Read the model definition and answer for the solid it produces. Units are mm, in the model's axes. Face numbers are marked on the shaded views. Coordinates: 2 decimals unless noted, no trailing zeros. Loops run counter-clockwise (first coordinate to the right, second up) from the corner with the lowest first, then second, coordinate; pieces in that order, holes last. Notation, with made-up numbers: M 69.5,9.5 L 124.5,9.5 A23 ccw 124.5,23.5 Z; hole C 59,-22 d6. An arc over 180 degrees is marked long. Put each result on its own line as item: value.
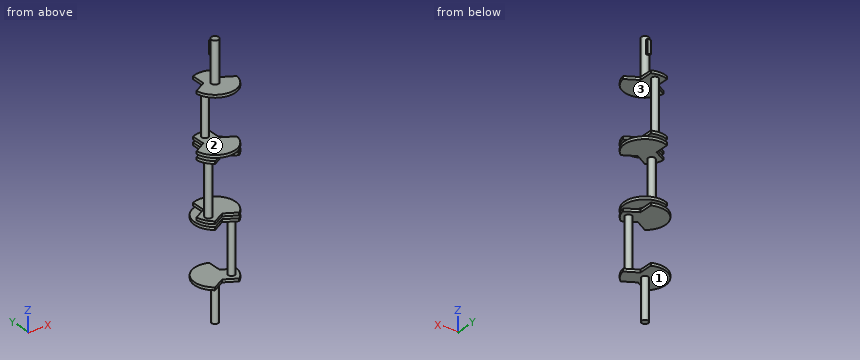
from build123d import *

# Parameters (mm, degrees)
BOSS_EXTRUDE1_DEPTH      = 5.08
LPATTERN1_COUNT          = 2
LPATTERN1_PITCH          = 104.14
BOSS_EXTRUDE2_REACH      = 119.176
SKETCH3_R                = 6.35
LPATTERN2_COUNT          = 3
LPATTERN2_PITCH          = 114.3
BODY_MOVE_COPY2_ANGLE    = 120
BODY_MOVE_COPY3_ANGLE    = 120
BOSS_EXTRUDE3_REACH      = 236.864
SKETCH5_R                = 12.7
BOSS_EXTRUDE4_START      = 114.3
SKETCH5_2_R              = 12.7
BOSS_EXTRUDE4_DEPTH      = 5.08
SKETCH6_R                = 6.985
BOSS_EXTRUDE5_DEPTH      = 76.2
SKETCH7_R                = 6.35
BOSS_EXTRUDE6_DEPTH      = 76.2
BOSS_EXTRUDE7_REACH      = 424.634
BOSS_EXTRUDE7_END_RADIUS = 6.985
BOSS_EXTRUDE7_START      = 10.16
SKETCH8_W                = 6.35
SKETCH8_H                = 25.4


with BuildPart() as part:
    # Sketch2 → Boss-Extrude1 (new body)
    with BuildSketch(Plane.XY):
        with BuildLine():
            Line((15.24, 8.798818102), (15.24, 34.919226796))
            ThreePointArc((15.24, 34.919226796), (0, 38.1), (-15.24, 34.919226796))
            Line((-15.24, 34.919226796), (-15.24, 8.798818102))
            Line((-15.24, 8.798818102), (-37.860937485, -4.261386244))
            ThreePointArc((-37.860937485, -4.261386244), (0, -38.1), (37.860937485, -4.261386244))
            Line((37.860937485, -4.261386244), (15.24, 8.798818102))
        make_face()
    extrude(amount=-BOSS_EXTRUDE1_DEPTH)


with BuildPart() as lpattern1_1:
    # LPattern1: pattern copy
    add(part.part.moved(Location(Vector(0, 0, 1) * (1 * LPATTERN1_PITCH))))

    # Sketch3 → Boss-Extrude2 (add, up to next)
    with BuildSketch(Plane.XY, mode=Mode.PRIVATE) as boss_extrude2_sk1:
        with Locations((0, 25.038762276)):
            Circle(SKETCH3_R)
    boss_extrude2_tool1 = extrude(boss_extrude2_sk1.sketch, amount=BOSS_EXTRUDE2_REACH, mode=Mode.PRIVATE) - lpattern1_1.part

    add(part.part)  # Boss-Extrude2 merges part
    add(boss_extrude2_tool1.solids().sort_by_distance((0, 25.038762, 0))[0])


with BuildPart() as lpattern2_1:
    # LPattern2: pattern copy
    add(lpattern1_1.part.moved(Location(Vector(0, 0, 1) * (1 * LPATTERN2_PITCH))))


with BuildPart() as lpattern2_2:
    # LPattern2: pattern copy
    add(lpattern1_1.part.moved(Location(Vector(0, 0, 1) * (2 * LPATTERN2_PITCH))))


with BuildPart() as lpattern2_1_1:
    # Body-Move/Copy2: moved
    add(lpattern2_1.part.rotate(Axis((0, -0.157266766, 0), (0, 0, 1)), BODY_MOVE_COPY2_ANGLE))

    # Sketch5 → Boss-Extrude3 (add, up to next)
    with BuildSketch(Plane.XY.offset(104.14), mode=Mode.PRIVATE) as boss_extrude3_sk1:
        Circle(SKETCH5_R)
    boss_extrude3_tool1 = extrude(boss_extrude3_sk1.sketch, amount=BOSS_EXTRUDE3_REACH, mode=Mode.PRIVATE) - lpattern2_1_1.part


with BuildPart() as lpattern1_1_1:
    # Body-Move/Copy3: moved
    add(lpattern1_1.part.rotate(Axis((0, 0, 0), (0, 0, -1)), BODY_MOVE_COPY3_ANGLE))


with BuildPart() as lpattern2_1_2:
    add(lpattern2_1_1.part)

    add(lpattern1_1_1.part)  # Boss-Extrude3 merges LPattern1_1
    add(boss_extrude3_tool1.solids().sort_by_distance((0, 0, 104.14))[0])


    add(lpattern2_2.part)  # Boss-Extrude4 merges LPattern2_2
    # Sketch5<2> → Boss-Extrude4 (add)
    with BuildSketch(Plane.XY.offset(104.14).offset(BOSS_EXTRUDE4_START)):
        with Locations(Location((0, 0, 0), (0, 0, 180))):
            Circle(SKETCH5_2_R)
    extrude(amount=BOSS_EXTRUDE4_DEPTH)

    # Sketch6 → Boss-Extrude5 (add)
    with BuildSketch(Plane.XY.offset(332.74)):
        with Locations(Location((0, 0, 0), (0, 0, 180))):
            Circle(SKETCH6_R)
    extrude(amount=BOSS_EXTRUDE5_DEPTH)

    # Sketch7 → Boss-Extrude6 (add)
    with BuildSketch(Plane(origin=(0, 0, -5.08), x_dir=(-1, 0, 0), z_dir=(0, 0, -1))):
        with Locations(Location((0, 0, 0), (0, 0, 180))):
            Circle(SKETCH7_R)
    extrude(amount=BOSS_EXTRUDE6_DEPTH)

    # Boss-Extrude7: up to this cylinder (the profile starts outside it)
    boss_extrude7_end = Plane(origin=(0, 0, 389.89), z_dir=(0, 0, -1)) * Cylinder(BOSS_EXTRUDE7_END_RADIUS, 864.238, mode=Mode.PRIVATE)
    # Sketch8 → Boss-Extrude7 (add, up to the surface)
    with BuildSketch(Plane(origin=(0, 0, 0), x_dir=(1, 0, 0), z_dir=(0, 1, 0)).offset(BOSS_EXTRUDE7_START), mode=Mode.PRIVATE) as boss_extrude7_sk1:
        with Locations((0, -389.89)):
            Rectangle(SKETCH8_W, SKETCH8_H)
    boss_extrude7_tool1 = extrude(boss_extrude7_sk1.sketch, amount=-BOSS_EXTRUDE7_REACH, mode=Mode.PRIVATE) - boss_extrude7_end
    add(boss_extrude7_tool1.solids().sort_by_distance((0, 10.16, 389.89))[0])


solid = lpattern2_1_2.part
1) Straight lines are drawn through the part: line 1 (Z direction, x = 13, y = 2); line 2 (Z direction, x = -33.5, y = 17); line 3 (X direction, y = -28, z = 114). For each, find the intervals that lie inside material, in ascending order. Write a range as [from, to].
Answer list:
line 1: z = [-5.08, 0], [99.06, 104.14], [109.22, 114.3], [213.36, 218.44], [223.52, 228.6], [327.66, 332.74]
line 2: z = [-5.08, 0], [99.06, 104.14]
line 3: x = [-26.23, -17.75], [17.47, 25.96]
2) Find section C-C, the plane z = 192.5. Write down the section's boundary in (x, y), plus the area to 3 significant figures.
Answer list:
outline: C -21.82,-12.76 d12.7
area: 127 mm^2
3) Given pin 1 Ø2 at (y, z) = (9, 387.5) entering from +X (3 decimals); pin 2 Ø12 at (x, y) = (25, 13.5) entering from -Z; pin 3 Ø1.5 at (y, z) = (23, 331.5) entering from -X, each flat-ended and moving along its own axis, determine where each tip first touches the part or whether it passes through.
Answer list:
pin 1: stops at x = 3.175
pin 2: stops at z = 109.22
pin 3: stops at x = -15.24
4) Determine the mould class of the marked faces 1, 2 and 3 for opening direction Z: released by +Z, released by -Z, zero draft, split by the parting line, or undercut.
Answer list:
face 1: released by -Z
face 2: undercut
face 3: undercut
5) Find section B-B, the plane y = 0. Count the separate pieces of the cut face and the enclosed holes in it, plus the area to 3 significant figures.
Answer list:
separate pieces: 4
enclosed holes: 0
area: 4,300 mm^2
6) Find section A-A, the plane z = 361. Write down the section's boundary in (x, y) (3 decimals), plus the area to 3 significant figures.
Answer list:
outline: C 0,0 d13.97
area: 153 mm^2
